Build history of the part. All positions in model axes, mm. Round coordinates to 2 decimals unless told otherwise and drop trailing zeros. Loops run counter-clockwise (first coordinate to the right, second up) from the corner with the lowest first, then second, coordinate; pieces in that order, holes last. Notation, with made-up numbers: (58, 81) - (108, 81) arc R31 cw to (108, 120) - close; hole circle Ø9 at (74, 25.5). An arc over 180 degrees is marked (long way). Use one line per item in the form item = value. Start each with the question number.
Q1. Saw through at B-B (z = 6.5). Give the cut face in (x, y) (3 decimals).
Q2. Saw through at A-A (x = 0). Give the cut face in (y, z) (3 decimals), then the cut area to 3 significant figures.
Q3. Pin check, flat tips, straight feed: pin 1 (5 mm diameter, centred on x = 13, z = 5, fed in from -Y); pin 2 (1.5 mm diameter, centred on y = -23, z = 3.5, fed in from +X); pin 3 (3.5 mm diameter, centred on x = 2, y = 1.5, fed in from -Z). Stop position of each tip, or through.
Q4. Drill centre lines: line 1 (Y direction, x = 0, z = 6.35) (3 decimals); line 2 (Y direction, x = 0, z = 3.2); line 3 (Y direction, x = -8.5, z = 5.75). Where is each one in solid material? Low to high.
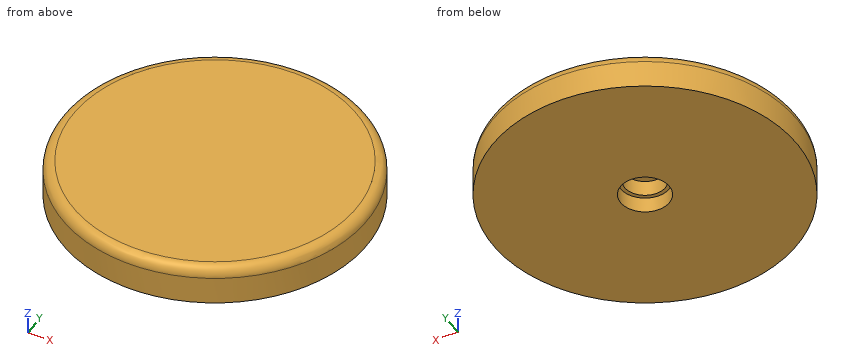
```python
from build123d import *

# Parameters (mm, degrees)
CROQUIS1_R              = 43.5901732
SALIENTE_EXTRUIR1_DEPTH = 11
REDONDEO1_R             = 3
CROQUIS2_R              = 5.875
CORTAR_EXTRUIR1_DEPTH   = 9
CROQUIS3_R              = 7
CORTAR_EXTRUIR2_DEPTH   = 4.5


with BuildPart() as part:
    # Croquis1 → Saliente-Extruir1 (new body)
    with BuildSketch(Plane.XY):
        Circle(CROQUIS1_R)
    extrude(amount=SALIENTE_EXTRUIR1_DEPTH)

    # Redondeo1
    redondeo1_edges = [part.edges().sort_by_distance(p)[0] for p in [
        (-43.5901732, 0, 11),
    ]]
    fillet(redondeo1_edges, radius=REDONDEO1_R)

    # Croquis2 → Cortar-Extruir1 (cut)
    with BuildSketch(Plane(origin=(0, 0, 0), x_dir=(-1, 0, 0), z_dir=(0, 0, -1))):
        Circle(CROQUIS2_R)
    extrude(amount=-CORTAR_EXTRUIR1_DEPTH, mode=Mode.SUBTRACT)

    # Croquis3 → Cortar-Extruir2 (cut)
    with BuildSketch(Plane(origin=(0, 0, 0), x_dir=(-1, 0, 0), z_dir=(0, 0, -1))):
        Circle(CROQUIS3_R)
    extrude(amount=-CORTAR_EXTRUIR2_DEPTH, mode=Mode.SUBTRACT)


solid = part.part
```
Report:
q1.outline = circle Ø87.18 at (0, 0); hole circle Ø11.75 at (0, 0)
q2.outline = (-43.59, 0) - (-7, 0) - (-7, 4.5) - (-5.875, 4.5) - (-5.875, 9) - (5.875, 9) - (5.875, 4.5) - (7, 4.5) - (7, 0) - (43.59, 0) - (43.59, 8) arc R3 ccw to (40.59, 11) - (-40.59, 11) arc R3 ccw to (-43.59, 8) - close
q2.area = 839 mm²
q3.pin_1 = -42.31
q3.pin_2 = 37.48
q3.pin_3 = 9
q4.line_1 = -43.59 to -5.875, 5.875 to 43.59
q4.line_2 = -43.59 to -7, 7 to 43.59
q4.line_3 = -42.75 to 42.75
